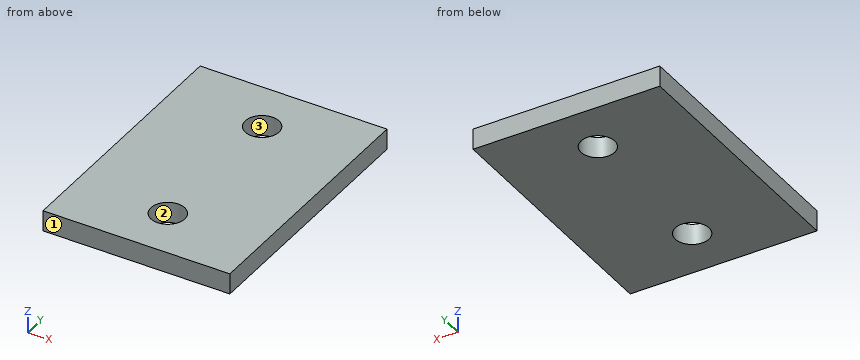
Autodesk Inventor part; units mm, degrees
ref_plane "YZ Plane" through (0, 0, 0) normal (1, 0, 0) x (0, 1, 0)
ref_plane "XZ Plane" through (0, 0, 0) normal (0, 1, 0) x (-1, 0, 0)
ref_plane "XY Plane" through (0, 0, 0) normal (0, 0, 1) x (1, 0, 0)
sketch "Sketch1" plane through (0, 0, 0) normal (0, 0, 1) x (1, 0, 0)
  line L0 (-9, -12.5) -> (9, -12.5)
  line L1 (9, -12.5) -> (9, 12.5)
  line L2 (9, 12.5) -> (-9, 12.5)
  line L3 (-9, 12.5) -> (-9, -12.5)
extrude "Extrusion1" add sketch "Sketch1" along normal blind 2
sketch "Sketch4" plane through (0, 0, 2) normal (0, 0, 1) x (1, 0, 0)
  circle A0 centre (0, 7.5) radius 1.625
  circle A1 centre (0, -7.5) radius 1.625
  point P0 (0, 0)
  dimension "d4" = 3.25
hole "Hole1" at (0, -7.5, 2) at (0, 7.5, 2) direction (0, 0, -1) diameter 3.25 end through all
properties part number "CONNECTOR_PLATE"
Source: CAD feature listing. Evaluate the final solid. Frame: model axes, mm. Face numbers are marked on the shaded views. Coordinates: 2 decimals unless noted, no trailing zeros. Write each loop counter-clockwise with the first axis right and the second up, starting at its lowest first coordinate (ties: lowest second). Pieces come first, ordered by that corner, then holes. Notation, with made-up numbers: (4.5, 55) -> (53.5, 55) arc R10 ccw to (53.5, 71) -> close; hole circle Ø2 at (21.5, 88). An arc over 180 degrees is marked (long way). Return JSON: item names as keys, results as strings. Group by question number.
1) Ray query, line 1 along Y through (x, z) = (0, 0.55) (3 decimals); line 2 along X through (y, z) = (7.5, 0.9) (3 decimals); line 3 along X through (y, z) = (6.5, 0.25). Return the intervals inside material, ascending.
2) Section query D-D, the plane y = -7. Return loops of the section in (x, z).
3) Section query C-C, the plane z = 0.6. Return loops of the section in (x, y) (3 decimals).
4) Section query A-A, the plane y = 7.5. Return loops of the section in (x, z) (3 decimals), plus the area to 3 significant figures.
5) Contact query for a flat-ended pin moving along its axis: P1, Ø3, axis at x = 0, y = -7.5, coming from the -Z side (3 decimals). Output: stop coordinate, or through.
6) Mould query, pull axis X, two halves, no side actions, for the marked faces 1, 2 and 3. Classes: +X half, -X half, draft (parallel to the pull), parting line (faces both ways), or undercut.
7) Section query B-B, the plane x = 0. Return loops of the section in (y, z) (3 decimals), plus the area to 3 significant figures.
From the geometry:
{
 "1": {"line 1": "-12.5 to -9.125, -5.875 to 5.875, 9.125 to 12.5", "line 2": "-9 to -1.625, 1.625 to 9", "line 3": "-9 to -1.28, 1.28 to 9"},
 "2": {"outline": "(-9, 0) -> (-1.55, 0) -> (-1.55, 2) -> (-9, 2) -> close; (1.55, 0) -> (9, 0) -> (9, 2) -> (1.55, 2) -> close"},
 "3": {"outline": "(-9, -12.5) -> (9, -12.5) -> (9, 12.5) -> (-9, 12.5) -> close; hole circle Ø3.25 at (0, -7.5); hole circle Ø3.25 at (0, 7.5)"},
 "4": {"outline": "(-9, 0) -> (-1.625, 0) -> (-1.625, 2) -> (-9, 2) -> close; (1.625, 0) -> (9, 0) -> (9, 2) -> (1.625, 2) -> close", "area": "29.5 mm²"},
 "5": {"P1": "through"},
 "6": {"face 1": "draft", "face 2": "undercut", "face 3": "undercut"},
 "7": {"outline": "(-12.5, 0) -> (-9.125, 0) -> (-9.125, 2) -> (-12.5, 2) -> close; (-5.875, 0) -> (5.875, 0) -> (5.875, 2) -> (-5.875, 2) -> close; (9.125, 0) -> (12.5, 0) -> (12.5, 2) -> (9.125, 2) -> close", "area": "37.0 mm²"}
}
